Geometry: final body of the model. Coordinates: model frame, mm. A direction names the side the tool comes from. Give positions to 0.01 mm unless a question says otherwise; leave off trailing zeros. Order: outer loops, then holes, each group sorted by start corner. A loop starts at its lowest first (then second) coordinate and runs counter-clockwise, first axis right, second up. Notation, with made-up numbers: (74, 32.5) -> (95, 32.5) arc R20 cw to (95, 36.5) -> close; hole circle Ø11 at (30, 71). An arc over 180 degrees is marked (long way). Answer in a Markdown table with one row per item. Add a question column.
Q1. Contact query for flat-ended pins moving along their axis: P1, Ø8, axis at y = 37, z = -5, coming from the -X side; P2, Ø8, axis at x = -137, z = -0.5, coming from the -Y side; P3, Ø1, axis at y = 56.5, z = 0, coming from the -X side; P4, Ø2.5, axis at x = -104.1, y = 0.47, coming from the -Z side. Output: stop coordinate, or through.
Q2. Pull-direction query (Y, two-part tool) for faces 1 (the face through (-193.249, -3.627, 1.479)), 2 (the face through (-129.6, 76, 1.5)), 3 (the face through (-123.105, 2, 1)); classes: +Y half, -Y half, draft (parallel to the pull), parting line (faces both ways), or undercut.
Q3. Cut plane C-C on x = -152. Return the cut outline in (y, z).
Q4. Set-up query: faces 4 (the face through (-178.01, 16.53, 1.48)), 5 (the face through (-104, 0, 0)), 6 (the face through (-167.861, 27.305, 1.479)), 7 (the face through (-100.007, 84.326, 1.479)), 8 (the face through (-106, 91, -23)). Return all of +Z, -Z, +X, -X, +Y, -Y with unobstructed straight access to the full face (end or side cutting, diameter ignored); none if empty.
Q5. Cut plane B-B on y = 46. Return the cut outline in (x, z).
Q6. Cut plane A-A on z = -7.5. Return the cut outline in (x, y), and give its area (3 significant figures).
Q7. Line query: line 1 along Z through (x, y) = (-130, 70); line 2 along X through (y, z) = (50, 1.25); line 3 along X through (y, z) = (90, -3.5). Output: solid intervals per line, ascending. Write a range as from..to.
Q8. Cut plane D-D on x = -142. Return the cut outline in (y, z).
from build123d import *

# Parameters (mm, degrees)
SALIENTE_EXTRUIR1_DEPTH = 3
CROQUIS2_R              = 3.5
CROQUIS2_R_2            = 1.5
SALIENTE_EXTRUIR2_DEPTH = 23
CROQUIS3_R              = 2
CORTAR_EXTRUIR1_DEPTH   = 3


with BuildPart() as part:
    # Croquis1 → Saliente-Extruir1 (new body)
    with BuildSketch(Plane.XY):
        with BuildLine():
            Line((-194.10496046, 92.470884256), (-194.10496046, 88.470884256))
            ThreePointArc((-194.10496046, 88.470884256), (-193.226280804, 86.349563912), (-191.10496046, 85.470884256))
            Line((-191.10496046, 85.470884256), (-188.10496046, 85.470884256))
            ThreePointArc((-188.10496046, 85.470884256), (-185.983640117, 84.592204599), (-185.10496046, 82.470884256))
            Line((-185.10496046, 82.470884256), (-185.10496046, 20.382772077))
            ThreePointArc((-185.10496046, 20.382772077), (-184.226280804, 18.261451734), (-182.10496046, 17.382772077))
            Line((-182.10496046, 17.382772077), (-180.10496046, 17.382772077))
            ThreePointArc((-180.10496046, 17.382772077), (-177.983640117, 16.504092421), (-177.10496046, 14.382772077))
            Line((-177.10496046, 14.382772077), (-177.10496046, 11.382772077))
            ThreePointArc((-177.10496046, 11.382772077), (-177.983640117, 9.261451734), (-180.10496046, 8.382772077))
            Line((-180.10496046, 8.382772077), (-191.10496046, 8.382772077))
            ThreePointArc((-191.10496046, 8.382772077), (-193.226280804, 7.504092421), (-194.10496046, 5.382772077))
            Line((-194.10496046, 5.382772077), (-194.10496046, -1.529115744))
            ThreePointArc((-194.10496046, -1.529115744), (-193.226280804, -3.650436088), (-191.10496046, -4.529115744))
            Line((-191.10496046, -4.529115744), (-165.10496046, -4.529115744))
            ThreePointArc((-165.10496046, -4.529115744), (-162.983640117, -3.650436088), (-162.10496046, -1.529115744))
            Line((-162.10496046, -1.529115744), (-162.10496046, 5.470884256))
            ThreePointArc((-162.10496046, 5.470884256), (-161.226280804, 7.592204599), (-159.10496046, 8.470884256))
            Line((-159.10496046, 8.470884256), (-126.10496046, 8.470884256))
            ThreePointArc((-126.10496046, 8.470884256), (-123.983640117, 7.592204599), (-123.10496046, 5.470884256))
            Line((-123.10496046, 5.470884256), (-123.10496046, -1.529115744))
            ThreePointArc((-123.10496046, -1.529115744), (-122.226280804, -3.650436088), (-120.10496046, -4.529115744))
            Line((-120.10496046, -4.529115744), (-102.10496046, -4.529115744))
            ThreePointArc((-102.10496046, -4.529115744), (-99.983640117, -3.650436088), (-99.10496046, -1.529115744))
            Line((-99.10496046, -1.529115744), (-99.10496046, 22.470884256))
            ThreePointArc((-99.10496046, 22.470884256), (-99.983640117, 24.592204599), (-102.10496046, 25.470884256))
            Line((-102.10496046, 25.470884256), (-111.10496046, 25.470884256))
            ThreePointArc((-111.10496046, 25.470884256), (-113.226280804, 26.349563912), (-114.10496046, 28.470884256))
            Line((-114.10496046, 28.470884256), (-114.10496046, 60.470884256))
            ThreePointArc((-114.10496046, 60.470884256), (-114.983640117, 62.592204599), (-117.10496046, 63.470884256))
            Line((-117.10496046, 63.470884256), (-118.10496046, 63.470884256))
            ThreePointArc((-118.10496046, 63.470884256), (-120.226280804, 64.349563912), (-121.10496046, 66.470884256))
            Line((-121.10496046, 66.470884256), (-121.10496046, 80.470884256))
            ThreePointArc((-121.10496046, 80.470884256), (-120.226280804, 82.592204599), (-118.10496046, 83.470884256))
            Line((-118.10496046, 83.470884256), (-102.10496046, 83.470884256))
            ThreePointArc((-102.10496046, 83.470884256), (-99.983640117, 84.349563912), (-99.10496046, 86.470884256))
            Line((-99.10496046, 86.470884256), (-99.10496046, 92.470884256))
            ThreePointArc((-99.10496046, 92.470884256), (-99.983640117, 94.592204599), (-102.10496046, 95.470884256))
            Line((-102.10496046, 95.470884256), (-191.10496046, 95.470884256))
            ThreePointArc((-191.10496046, 95.470884256), (-193.226280804, 94.592204599), (-194.10496046, 92.470884256))
        make_face()
        with BuildLine():
            Line((-165.422187349, 50.715677144), (-181.973694619, 50.715677144))
            ThreePointArc((-181.973694619, 50.715677144), (-167.512513703, 27.100940434), (-139.830961352, 26.384558748))
            Line((-139.830961352, 26.384558748), (-148.106714986, 40.718584514))
            ThreePointArc((-148.106714986, 40.718584514), (-159.262513703, 41.390359596), (-165.422187349, 50.715677144))
        make_face(mode=Mode.SUBTRACT)
        with BuildLine():
            Line((-165.422187349, 53.715677144), (-181.973694619, 53.715677144))
            ThreePointArc((-181.973694619, 53.715677144), (-167.512513703, 77.330413853), (-139.830961352, 78.04679554))
            Line((-139.830961352, 78.04679554), (-148.106714986, 63.712769774))
            ThreePointArc((-148.106714986, 63.712769774), (-159.262513703, 63.040994691), (-165.422187349, 53.715677144))
        make_face(mode=Mode.SUBTRACT)
        with BuildLine():
            Line((-145.508638775, 62.212769774), (-137.23288514, 76.54679554))
            ThreePointArc((-137.23288514, 76.54679554), (-124.012513703, 52.215677144), (-137.23288514, 27.884558748))
            Line((-137.23288514, 27.884558748), (-145.508638775, 42.218584514))
            ThreePointArc((-145.508638775, 42.218584514), (-140.512513703, 52.215677144), (-145.508638775, 62.212769774))
        make_face(mode=Mode.SUBTRACT)
    extrude(amount=SALIENTE_EXTRUIR1_DEPTH)

    # Croquis2 → Saliente-Extruir2 (add)
    with BuildSketch(Plane(origin=(0, 0, 0), x_dir=(-1, 0, 0), z_dir=(0, 0, -1))):
        with Locations((189.10496046, 90.470884256)):
            Circle(CROQUIS2_R)
        with Locations((189.10496046, 90.470884256)):
            Circle(CROQUIS2_R_2, mode=Mode.SUBTRACT)
        with Locations((104.10496046, 90.470884256)):
            Circle(CROQUIS2_R)
        with Locations((104.10496046, 90.470884256)):
            Circle(CROQUIS2_R_2, mode=Mode.SUBTRACT)
        with Locations((104.10496046, 0.470884256)):
            Circle(CROQUIS2_R)
        with Locations((104.10496046, 0.470884256)):
            Circle(CROQUIS2_R_2, mode=Mode.SUBTRACT)
        with Locations((189.10496046, 0.470884256)):
            Circle(CROQUIS2_R)
        with Locations((189.10496046, 0.470884256)):
            Circle(CROQUIS2_R_2, mode=Mode.SUBTRACT)
    extrude(amount=SALIENTE_EXTRUIR2_DEPTH)

    # Croquis3 → Cortar-Extruir1 (cut)
    with BuildSketch(Plane.XY.offset(3)):
        with Locations((-178.012513703, 77.215677144)):
            Circle(CROQUIS3_R)
        with Locations((-128.012513703, 77.215677144)):
            Circle(CROQUIS3_R)
        with Locations((-128.012513703, 27.215677144)):
            Circle(CROQUIS3_R)
        with Locations((-178.012513703, 27.215677144)):
            Circle(CROQUIS3_R)
    extrude(amount=-CORTAR_EXTRUIR1_DEPTH, mode=Mode.SUBTRACT)


solid = part.part
Completed:
| question | item | result |
|---|---|---|
| 1 | P1 | passes through |
| 1 | P2 | stops at y = 8.47 |
| 1 | P3 | stops at x = -185.1 |
| 1 | P4 | stops at z = 0 |
| 2 | face 1 | -Y half |
| 2 | face 2 | undercut |
| 2 | face 3 | draft |
| 3 | outline | (8.47, 0) -> (23.23, 0) -> (23.23, 3) -> (8.47, 3) -> close; (39.76, 0) -> (64.67, 0) -> (64.67, 3) -> (39.76, 3) -> close; (81.2, 0) -> (95.47, 0) -> (95.47, 3) -> (81.2, 3) -> close |
| 4 | face 4 | +Z, -Z, -X |
| 4 | face 5 | -Z |
| 4 | face 6 | +Z, -Z |
| 4 | face 7 | +Z, -Z, +X |
| 4 | face 8 | -Z, +X, -X, +Y, -Y |
| 5 | outline | (-185.1, 0) -> (-181.34, 0) -> (-181.34, 3) -> (-185.1, 3) -> close; (-163.86, 0) -> (-142.17, 0) -> (-142.17, 3) -> (-163.86, 3) -> close; (-124.69, 0) -> (-114.1, 0) -> (-114.1, 3) -> (-124.69, 3) -> close |
| 6 | outline | circle Ø7 at (-189.1, 0.47); circle Ø7 at (-189.1, 90.47); circle Ø7 at (-104.1, 0.47); circle Ø7 at (-104.1, 90.47); hole circle Ø3 at (-189.1, 0.47); hole circle Ø3 at (-189.1, 90.47); hole circle Ø3 at (-104.1, 0.47); hole circle Ø3 at (-104.1, 90.47) |
| 6 | area | 126 mm² |
| 7 | line 1 | z = 0..3 |
| 7 | line 2 | x = -185.1..-181.93, -165.31..-140.71, -124.1..-114.1 |
| 7 | line 3 | x = -192.57..-190.53, -187.68..-185.64, -107.57..-105.53, -102.68..-100.64 |
| 8 | outline | (8.47, 0) -> (25.39, 0) -> (25.39, 3) -> (8.47, 3) -> close; (30.14, 0) -> (36.14, 0) -> (36.14, 3) -> (30.14, 3) -> close; (46.3, 0) -> (58.13, 0) -> (58.13, 3) -> (46.3, 3) -> close; (68.29, 0) -> (74.29, 0) -> (74.29, 3) -> (68.29, 3) -> close; (79.04, 0) -> (95.47, 0) -> (95.47, 3) -> (79.04, 3) -> close |
